Source: CAD feature listing. Evaluate the final solid. Frame: model axes, mm. Round coordinates to 2 decimals unless told otherwise and drop trailing zeros. Order: outer loops, then holes, each group sorted by start corner. A loop starts at its lowest first (then second) coordinate and runs counter-clockwise, first axis right, second up. Notation, with made-up numbers: (71, 83) -> (79, 83) arc R30 cw to (79, 107) -> close; hole circle Ø5 at (36.5, 65). An arc over 180 degrees is marked (long way). One line per item, written item: value. Start each with the question number.
1) Ray query, L1, parallel to Y at x = 2.5, z = -0.05; L2, parallel to Z at x = 7, y = 4. Return the intervals inside material, ascending.
2) Section A-A (x = 4.5). Return the cut outline in (y, z), and give its area (3 significant figures).
3) Section B-B (y = 1.15). Return the cut outline in (x, z), and give its area (3 significant figures).
4) Mould query, pull axis X, two halves, no side actions, for faces 1 (the face through (4, 4, 0)), 2 (the face through (4, 3, 0.5)). Classes: pulls with the +X half, pulls with the -X half, needs draft (parallel to the pull), parting line crosses it, or undercut.
5) Section C-C (x = 6). Return the cut outline in (y, z).
```python
from build123d import *

# Parameters (mm, degrees)
F0_W     = 9
F0_H     = 6
F1_DEPTH = 0.5
F2_R     = 0.25
F3_DEPTH = 0.2


with BuildPart() as f1:
    # F0 (on Top) → F1 (new body)
    with BuildSketch(Plane.XY):
        with Locations((4.5, 3)):
            Rectangle(F0_W, F0_H)
    extrude(amount=F1_DEPTH)

    # F2 (on face) → F3 (join)
    with BuildSketch(Plane(origin=(0, 0, 0), x_dir=(1, 0, 0), z_dir=(0, 0, -1))):
        with Locations((0.5, -0.5)):
            Circle(F2_R)
        with Locations((1.5, -0.5)):
            Circle(F2_R)
        with Locations((2.5, -0.5)):
            Circle(F2_R)
        with Locations((3.5, -0.5)):
            Circle(F2_R)
        with Locations((4.5, -0.5)):
            Circle(F2_R)
        with Locations((5.5, -0.5)):
            Circle(F2_R)
        with Locations((6.5, -0.5)):
            Circle(F2_R)
        with Locations((7.5, -0.5)):
            Circle(F2_R)
        with Locations((8.5, -0.5)):
            Circle(F2_R)
        with Locations((8.5, -1.5)):
            Circle(F2_R)
        with Locations((7.5, -1.5)):
            Circle(F2_R)
        with Locations((6.5, -1.5)):
            Circle(F2_R)
        with Locations((5.5, -1.5)):
            Circle(F2_R)
        with Locations((4.5, -1.5)):
            Circle(F2_R)
        with Locations((3.5, -1.5)):
            Circle(F2_R)
        with Locations((2.5, -1.5)):
            Circle(F2_R)
        with Locations((1.5, -1.5)):
            Circle(F2_R)
        with Locations((0.5, -1.5)):
            Circle(F2_R)
        with Locations((8.5, -2.5)):
            Circle(F2_R)
        with Locations((7.5, -2.5)):
            Circle(F2_R)
        with Locations((6.5, -2.5)):
            Circle(F2_R)
        with Locations((5.5, -2.5)):
            Circle(F2_R)
        with Locations((4.5, -2.5)):
            Circle(F2_R)
        with Locations((3.5, -2.5)):
            Circle(F2_R)
        with Locations((2.5, -2.5)):
            Circle(F2_R)
        with Locations((1.5, -2.5)):
            Circle(F2_R)
        with Locations((0.5, -2.5)):
            Circle(F2_R)
        with Locations((8.5, -3.5)):
            Circle(F2_R)
        with Locations((7.5, -3.5)):
            Circle(F2_R)
        with Locations((6.5, -3.5)):
            Circle(F2_R)
        with Locations((5.5, -3.5)):
            Circle(F2_R)
        with Locations((4.5, -3.5)):
            Circle(F2_R)
        with Locations((3.5, -3.5)):
            Circle(F2_R)
        with Locations((2.5, -3.5)):
            Circle(F2_R)
        with Locations((1.5, -3.5)):
            Circle(F2_R)
        with Locations((0.5, -3.5)):
            Circle(F2_R)
        with Locations((8.5, -4.5)):
            Circle(F2_R)
        with Locations((7.5, -4.5)):
            Circle(F2_R)
        with Locations((6.5, -4.5)):
            Circle(F2_R)
        with Locations((5.5, -4.5)):
            Circle(F2_R)
        with Locations((4.5, -4.5)):
            Circle(F2_R)
        with Locations((3.5, -4.5)):
            Circle(F2_R)
        with Locations((2.5, -4.5)):
            Circle(F2_R)
        with Locations((1.5, -4.5)):
            Circle(F2_R)
        with Locations((0.5, -4.5)):
            Circle(F2_R)
        with Locations((8.5, -5.5)):
            Circle(F2_R)
        with Locations((7.5, -5.5)):
            Circle(F2_R)
        with Locations((6.5, -5.5)):
            Circle(F2_R)
        with Locations((5.5, -5.5)):
            Circle(F2_R)
        with Locations((4.5, -5.5)):
            Circle(F2_R)
        with Locations((3.5, -5.5)):
            Circle(F2_R)
        with Locations((2.5, -5.5)):
            Circle(F2_R)
        with Locations((1.5, -5.5)):
            Circle(F2_R)
        with Locations((0.5, -5.5)):
            Circle(F2_R)
    extrude(amount=F3_DEPTH)


solid = f1.part
```
Findings:
1. L1: 0.25 to 0.75, 1.25 to 1.75, 2.25 to 2.75, 3.25 to 3.75, 4.25 to 4.75, 5.25 to 5.75
1. L2: 0 to 0.5
2. outline: (0, 0) -> (0.25, 0) -> (0.25, -0.2) -> (0.75, -0.2) -> (0.75, 0) -> (1.25, 0) -> (1.25, -0.2) -> (1.75, -0.2) -> (1.75, 0) -> (2.25, 0) -> (2.25, -0.2) -> (2.75, -0.2) -> (2.75, 0) -> (3.25, 0) -> (3.25, -0.2) -> (3.75, -0.2) -> (3.75, 0) -> (4.25, 0) -> (4.25, -0.2) -> (4.75, -0.2) -> (4.75, 0) -> (5.25, 0) -> (5.25, -0.2) -> (5.75, -0.2) -> (5.75, 0) -> (6, 0) -> (6, 0.5) -> (0, 0.5) -> close
2. area: 3.60 mm2
3. outline: (0, 0) -> (9, 0) -> (9, 0.5) -> (0, 0.5) -> close
3. area: 4.50 mm2
4. face 1: undercut
4. face 2: needs draft
5. outline: (0, 0) -> (6, 0) -> (6, 0.5) -> (0, 0.5) -> close
